Here's how the part is built. I have some questions about the finished solid (model axes, mm). A direction names the side the tool comes from. Coordinates: 2 decimals unless noted, no trailing zeros. Order: outer loops, then holes, each group sorted by start corner. A loop starts at its lowest first (then second) coordinate and runs counter-clockwise, first axis right, second up. Notation, with made-up numbers: (72.25, -23.5) - (116.25, -23.5) arc R13 ccw to (116.25, -14.5) - close; hole circle Ø9 at (63, -24.75). An arc over 180 degrees is marked (long way). Use CSV: the item, a comma, the result in double quotes. Start each with the question number.
Autodesk Inventor part; units mm, degrees
ref_plane "YZ Plane" through (0, 0, 0) normal (1, 0, 0) x (0, 1, 0)
ref_plane "XZ Plane" through (0, 0, 0) normal (0, 1, 0) x (-1, 0, 0)
ref_plane "XY Plane" through (0, 0, 0) normal (0, 0, 1) x (1, 0, 0)
sketch "Эскиз2" plane through (0, 0, 0) normal (0, 0, 1) x (1, 0, 0)
  line L0 (0, 0) -> (20, 0)
  line L1 (20, 0) -> (20, 3)
  line L2 (20, 3) -> (0, 3)
  line L3 (0, 3) -> (0, 0)
  dimension "d14" = 20
  dimension "d15" = 3
extrude "Выдавливание2" add sketch "Эскиз2" along normal mid plane 100
fillet "Сопряжение1" radius 4 2 edges at (0, 1.5, 50) (0, 1.5, -50)
sketch "Эскиз5" plane through (20, 3, 50) normal (0, 1, 0) x (1, 0, 0)
  line L0 (0, 100) -> (0, 0)
  line L1 (0, 0) -> (-16, 0)
  line L2 (0, 100) -> (-3.42, 100)
  line L3 (-3.42, 100) -> (-3.42, 0)
  line L4 (-3.42, 0) -> (0, 0)
  line L5 (0, 0) -> (0, 100)
  point P0 (-20, 50)
  dimension "d25" = 3.42
extrude "Выдавливание4" add sketch "Эскиз5" along normal blind 3
sketch "Эскиз6" plane through (0, 0, 50) normal (0, 0, 1) x (1, 0, 0)
  circle A0 centre (18.08, 4.5) radius 1
  line L0 (16.58, 6) -> (20, 6)
  line L1 (16.58, 3) -> (16.58, 6)
  point P0 (0, 0)
  dimension "d28" = 2
  dimension "d29" = 1.5
  dimension "d30" = 1.5
extrude "Выдавливание5" cut sketch "Эскиз6" against normal through all
sketch "Эскиз7" plane through (20, 6, 50) normal (0, 1, 0) x (1, 0, 0)
  line L0 (-3.42, 100) -> (-3.42, 0)
  line L1 (0, 0) -> (0, 100)
  line L2 (-3.42, 25) -> (0, 25)
  line L3 (0, 25) -> (0, 75)
  line L4 (0, 75) -> (-3.42, 75)
  line L5 (-3.42, 75) -> (-3.42, 25)
  line L6 (-3.42, 0) -> (-16, 0)
  point P0 (-20, 50)
  point P1 (-3.42, 75)
  point P2 (0, 25)
  dimension "d33" = 50
  dimension "d34" = 25
extrude "Выдавливание6" cut sketch "Эскиз7" against normal blind 3
fillet "Сопряжение2" radius 1.5 4 edges at (20, 6, 37.5) (16.58, 6, 37.5) (20, 6, -37.5) (16.58, 6, -37.5)
sketch "Эскиз8" plane through (16.58, 3, -25) normal (0, 0, 1) x (1, 0, 0)
  line L0 (3.42, -3) -> (3.42, 1.5)
  line L1 (0, 0.9343) -> (3.42, -3)
  line L2 (3.42, -3) -> (-12.58, -3)
  line L3 (0, 0) -> (0, 1.5)
  line L4 (0, 0.9343) -> (3.42, 0.9343)
  point P0 (-16.58, -3)
  dimension "d38" = 49
extrude "Выдавливание7" cut sketch "Эскиз8" along normal up to surface (50 mm away)
properties part number "Cover"
Item 1: Suppose I cut it at B-B on x = 9.25. Write out the boundary of the cut face in (y, z).
Item 2: Suppose I cut it at C-C on y = 1.75. Write out the boundary of the cut face in (x, z).
Item 3: For pin 1 Ø1.6 at (y, z) = (3.5, 39.5) entering from -X; pin 2 Ø1 at (x, z) = (7, 17.5) entering from +Y; pin 3 Ø0.8 at (y, z) = (3.5, -42.5) entering from -X, each with a flat end and sliding along its axis, tell me the tip position at first contact or that it passes through.
Item 4: For faces 1 (the cylindrical face through (17.343, 5.176, -37.325)), 2 (the flat face through (19, 3, -25)), which set-ups out of +Z, -Z, +X, -X, +Y, -Y let a thin tool reach every point of the face, with its end or its side?
Item 5: Suppose I cut it at A-A on z = -36.5. Write out the boundary of the cut face in (x, y), then the cut area to 3 significant figures.
Item 6: Please list where these lines run through material, in increasing order: line 1 along X through (y, z) = (4.5, -41.75); line 2 along Y through (x, z) = (18.08, -33.25); line 3 along Y through (x, z) = (13, -37.5). Write a range as from..to.
Item 7: Suppose I cut it at D-D on z = 20. Write out the boundary of the cut face in (x, y).
Item 8: We'd pull the mould along Z, two halves only. Please class faces 3 (the flat face through (12, 2, 50)), 4 (the flat face through (19, 3, 25)), 5 (the flat face through (12, 2, -50)): released by +Z, released by -Z, zero draft, split by the parting line, or undercut.
Here are the results:
1,outline,"(0, -50) - (3, -50) - (3, 50) - (0, 50) - close"
2,outline,"(0, -46) arc R4 ccw to (4, -50) - (20, -50) - (20, -25) - (18.48, -25) - (18.48, 25) - (20, 25) - (20, 50) - (4, 50) arc R4 ccw to (0, 46) - close"
3,pin 1,"x = 0"
3,pin 2,"y = 3"
3,pin 3,"x = 16.58"
4,face 1,"+Z, -Z"
4,face 2,"+X, +Y"
5,outline,"(0, 0) - (20, 0) - (20, 4.5) arc R1.5 ccw to (18.5, 6) - (18.08, 6) arc R1.5 ccw to (16.58, 4.5) - (16.58, 3) - (0, 3) - close; hole circle Ø2 at (18.08, 4.5)"
5,area,"66.2 mm^2"
6,line 1,"16.58..17.08, 19.08..20"
6,line 2,"0..3.5, 5.5..6"
6,line 3,"0..3"
7,outline,"(0, 0) - (20, 0) - (17.39, 3) - (0, 3) - close"
8,face 3,"released by +Z"
8,face 4,"undercut"
8,face 5,"released by -Z"
